```python
from build123d import *

# Parameters (mm, degrees)
F0_W      = 101.6
F0_H      = 101.6
F1_DEPTH  = 50.8
F2_R      = 44.45
F3_DEPTH  = 17.78
F4_R      = 44.45
F5_DEPTH  = 17.78
F6_R      = 44.45
F7_DEPTH  = 17.78
F8_R      = 44.45
F9_DEPTH  = 17.78
F10_R     = 44.45
F11_DEPTH = 17.78
F12_R     = 44.45
F13_DEPTH = 17.78


with BuildPart() as f1:
    # F0 (on Front) → F1 (new body, symmetric)
    with BuildSketch(Plane.XZ):
        Rectangle(F0_W, F0_H)
    extrude(amount=F1_DEPTH, both=True)

    # F2 (on face) → F3 (cut)
    with BuildSketch(Plane.XZ.offset(50.8)):
        Circle(F2_R)
    extrude(amount=-F3_DEPTH, mode=Mode.SUBTRACT)

    # F4 (on face) → F5 (cut)
    with BuildSketch(Plane(origin=(0, 0, -50.8), x_dir=(1, 0, 0), z_dir=(0, 0, -1))):
        Circle(F4_R)
    extrude(amount=-F5_DEPTH, mode=Mode.SUBTRACT)

    # F6 (on face) → F7 (cut)
    with BuildSketch(Plane.YZ.offset(50.8)):
        Circle(F6_R)
    extrude(amount=-F7_DEPTH, mode=Mode.SUBTRACT)

    # F8 (on face) → F9 (cut)
    with BuildSketch(Plane.XY.offset(50.8)):
        Circle(F8_R)
    extrude(amount=-F9_DEPTH, mode=Mode.SUBTRACT)

    # F10 (on face) → F11 (cut)
    with BuildSketch(Plane(origin=(0, 50.8, 0), x_dir=(-1, 0, 0), z_dir=(0, 1, 0))):
        Circle(F10_R)
    extrude(amount=-F11_DEPTH, mode=Mode.SUBTRACT)

    # F12 (on face) → F13 (cut)
    with BuildSketch(Plane(origin=(-50.8, 0, 0), x_dir=(0, -1, 0), z_dir=(-1, 0, 0))):
        Circle(F12_R)
    extrude(amount=-F13_DEPTH, mode=Mode.SUBTRACT)

    # F14 (on Front) → F15 (revolve)
    with BuildSketch(Plane.XZ):
        Polygon((-35.56, 33.02), (0, 33.02), (0, 83.82), align=None)
        Polygon((35.56, -33.02), (0, -33.02), (0, -83.82), align=None)
    revolve(axis=Axis((0, 0, -58.42), (0, 0, 1)))

    # F16 (on Front) → F17 (revolve)
    with BuildSketch(Plane.XZ):
        Polygon((-83.82, 0), (-33.02, 0), (-33.02, 35.56), align=None)
        Polygon((83.82, 0), (33.02, 0), (33.02, -35.56), align=None)
    revolve(axis=Axis((58.42, 0, 0), (-1, 0, 0)))

    # F18 (on Right) → F19 (revolve)
    with BuildSketch(Plane.YZ):
        Polygon((-83.82, 0), (-33.02, 0), (-33.02, 35.56), align=None)
        Polygon((83.82, 0), (33.02, 0), (33.02, -35.56), align=None)
    revolve(axis=Axis((0, 58.42, 0), (0, -1, 0)))


solid = f1.part
```
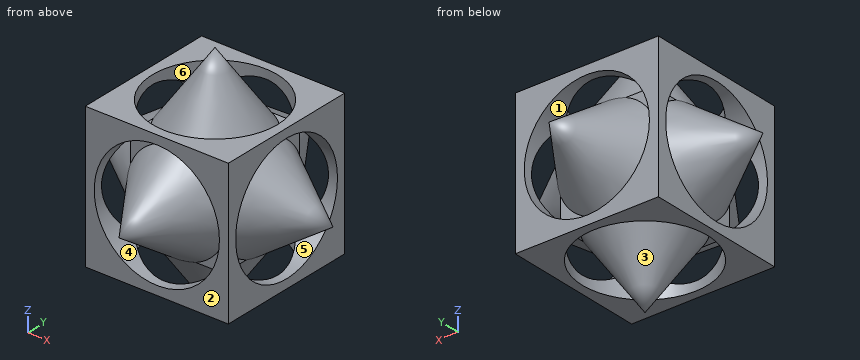
Check sheet for the modelled part. Datum: model origin and axes. Units: mm. Face numbers are marked on the shaded views. A direction names the side the tool comes from. Round coordinates to 2 decimals unless told otherwise and drop trailing zeros. Loops run counter-clockwise (first coordinate to the right, second up) from the corner with the lowest first, then second, coordinate; pieces in that order, holes last. Notation, with made-up numbers: (68.25, 15.5) -> (125.25, 15.5) arc R24 cw to (125.25, 37.5) -> close; hole circle Ø5 at (41, -6). An arc over 180 degrees is marked (long way). Answer in a Markdown table with one row per item.
Q1. Release check for a two-part mould opening along Z. For the marked faces 1, 2 and 3 record: released by +Z, released by -Z, zero draft, split by the parting line, or undercut.
Data:
| item | result |
|---|---|
| face 1 | undercut |
| face 2 | zero draft |
| face 3 | released by -Z |
Q2. Set-up check for the marked faces 4, 5 and 6: record each of +Z, -Z, +X, -X, +Y, -Y from which the full face is reachable in a straight line by a thin tool's end or side.
Data:
| item | result |
|---|---|
| face 4 | -Y |
| face 5 | +X |
| face 6 | +Z |
Q3. Sectioned sample at A-A on z = -41. Enter the section's corners in (x, y), then the cut area to 3 significant figures.
Data:
| item | result |
|---|---|
| outline | (-50.8, -50.8) -> (-17.17, -50.8) -> (-17.17, -41) arc R44.45 cw to (-41, -17.17) -> (-50.8, -17.17) -> close; (-50.8, 17.17) -> (-41, 17.17) arc R44.45 cw to (-17.17, 41) -> (-17.17, 50.8) -> (-50.8, 50.8) -> close; circle Ø59.95 at (0, 0); (17.17, -50.8) -> (50.8, -50.8) -> (50.8, -17.17) -> (41, -17.17) arc R44.45 cw to (17.17, -41) -> close; (17.17, 41) arc R44.45 cw to (41, 17.17) -> (50.8, 17.17) -> (50.8, 50.8) -> (17.17, 50.8) -> close |
| area | 5,910 mm^2 |
Q4. Thickness scan on L1, parallel to Z at x = 0, y = 46.25; L2, parallel to X at y = 39, z = -22.5 (3 decimals); L3, parallel to Y at x = -18, z = -45.5. Record the ranges inside material, lowest first.
Data:
| item | result |
|---|---|
| L1 | z = -50.8 to -44.45, -26.3 to 26.3, 44.45 to 50.8 |
| L2 | x = -50.8 to -38.335, -21.865 to 21.865, 38.335 to 50.8 |
| L3 | y = -50.8 to -40.64, -19.89 to 19.89, 40.64 to 50.8 |
Q5. Go/stop test with flat-tipped pins: P1, Ø6, axis at x = -19, y = -20, coming from the +Z side; P2, Ø1, axis at x = -45.5, z = 7.5, coming from the +Y side; P3, Ø12, axis at x = -39.5, z = -13.5, coming from the -Y side. Record where each tip stops, or that it passes through.
Data:
| item | result |
|---|---|
| P1 | stops at z = 48.7 |
| P2 | stops at y = 50.8 |
| P3 | stops at y = -50.8 |
Q6. Sectioned sample at B-B on y = -9. Give the number of separate pieces and of enclosed holes in the cut face, then the cut area to 3 significant figures.
Data:
| item | result |
|---|---|
| separate pieces | 5 |
| enclosed holes | 0 |
| area | 10,600 mm^2 |
